For this review, take the finished solid that the model builds, in its own axes (mm). Face numbers are marked on the shaded views. A direction names the side the tool comes from. Round coordinates to 2 decimals unless told otherwise and drop trailing zeros. Order: outer loops, then holes, each group sorted by start corner. A loop starts at its lowest first (then second) coordinate and runs counter-clockwise, first axis right, second up. Notation, with made-up numbers: M 31,15 L 49,15 A17 ccw 49,32 Z; hole C 89,-21 d9. An arc over 180 degrees is marked long. Answer as a JSON object with one key per item and string values.
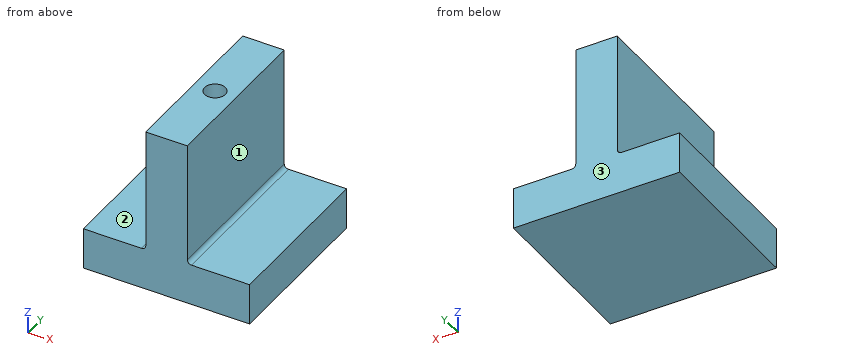
from build123d import *

# Parameters (mm, degrees)
F1_DEPTH = 20
F3_D     = 5
F3_DEPTH = 15.7
F3_TIP   = 1.5021515476
F4_R     = 1


with BuildPart() as f1:
    # F0 (on Front) → F1 (new body, symmetric)
    with BuildSketch(Plane.XZ):
        Polygon((5, 30), (-5, 30), (-5, 0), (-20, 0), (-20, -10), (20, -10), (20, 0), (5, 0), align=None)
    extrude(amount=F1_DEPTH, both=True)

    # F3
    with Locations(Plane.XY.offset(30)):
        with Locations((0, 0)):
            Hole(F3_D / 2, depth=F3_DEPTH)
            with Locations((0, 0, -(F3_DEPTH + F3_TIP / 2))):  # 118° drill point
                Cone(0, F3_D / 2, F3_TIP, mode=Mode.SUBTRACT)

    # F4
    f4_edges = [f1.edges().sort_by_distance(p)[0] for p in [
        (5, 0, 0),
        (-5, 0, 0),
    ]]
    fillet(f4_edges, radius=F4_R)


solid = f1.part
1) Machinability: for the marked faces 1, 2 and 3, which of the approach directions +Z, -Z, +X, -X, +Y, -Y give a long, thin tool a straight path to every point of the face, cutting with its end or side? Answer none if there is none.
Geometry check:
{"face 1": "+Z, +X, +Y, -Y", "face 2": "+Z, -X, +Y, -Y", "face 3": "+Z, -Z, +X, -X, +Y"}
2) For L1, parallel to Y at x = 0, z = 20; L2, parallel to X at y = 0, z = 25; L3, parallel to X at y = 13.5, z = 9.5, list the stretches that pass through material, from the lowest coordinate up.
Geometry check:
{"L1": "y = -20 to -2.5, 2.5 to 20", "L2": "x = -5 to -2.5, 2.5 to 5", "L3": "x = -5 to 5"}
3) Add section C-C on x = 13. State the section outline as (y, z) points, and give its area (3 significant figures).
Geometry check:
{"outline": "M -20,-10 L 20,-10 L 20,0 L -20,0 Z", "area": "400 mm²"}
4) Insertion check: P1, Ø14.5, axis at y = 2.5, z = 9, coming from the +X side; P2, Ø4, axis at x = -11.5, y = 2, coming from the +Z side; P3, Ø1.5, axis at y = -11.5, z = 1, coming from the +X side. Each pin has a flat end and moves straight along its axis. Give the tip position at first contact, or say it passes through.
Geometry check:
{"P1": "stops at x = 5", "P2": "stops at z = 0", "P3": "stops at x = 5.34"}
5) Add section A-A on y = 17. State the section outline as (x, z) points, and give its area (3 significant figures).
Geometry check:
{"outline": "M -20,-10 L 20,-10 L 20,0 L 6,0 A1 cw 5,1 L 5,30 L -5,30 L -5,1 A1 cw -6,0 L -20,0 Z", "area": "700 mm²"}
6) Add section D-D on z = 8. State the section outline as (x, y) points, and give its area (3 significant figures).
Geometry check:
{"outline": "M -5,-20 L 5,-20 L 5,20 L -5,20 Z", "area": "400 mm²"}
7) Add section B-B on z = 16. State the section outline as (x, y) points, and give its area (3 significant figures).
Geometry check:
{"outline": "M -5,-20 L 5,-20 L 5,20 L -5,20 Z; hole C 0,0 d5", "area": "380 mm²"}
